Geometry check sheet. Reference: drawing and pictorial views, mm from the part's lowest x, y, z. Round coordinates to 2 decimals unless told otherwise and drop trailing zeros. Order: outer loops, then holes, each group sorted by start corner. A loop starts at its lowest first (then second) coordinate and runs counter-clockwise, first axis right, second up.
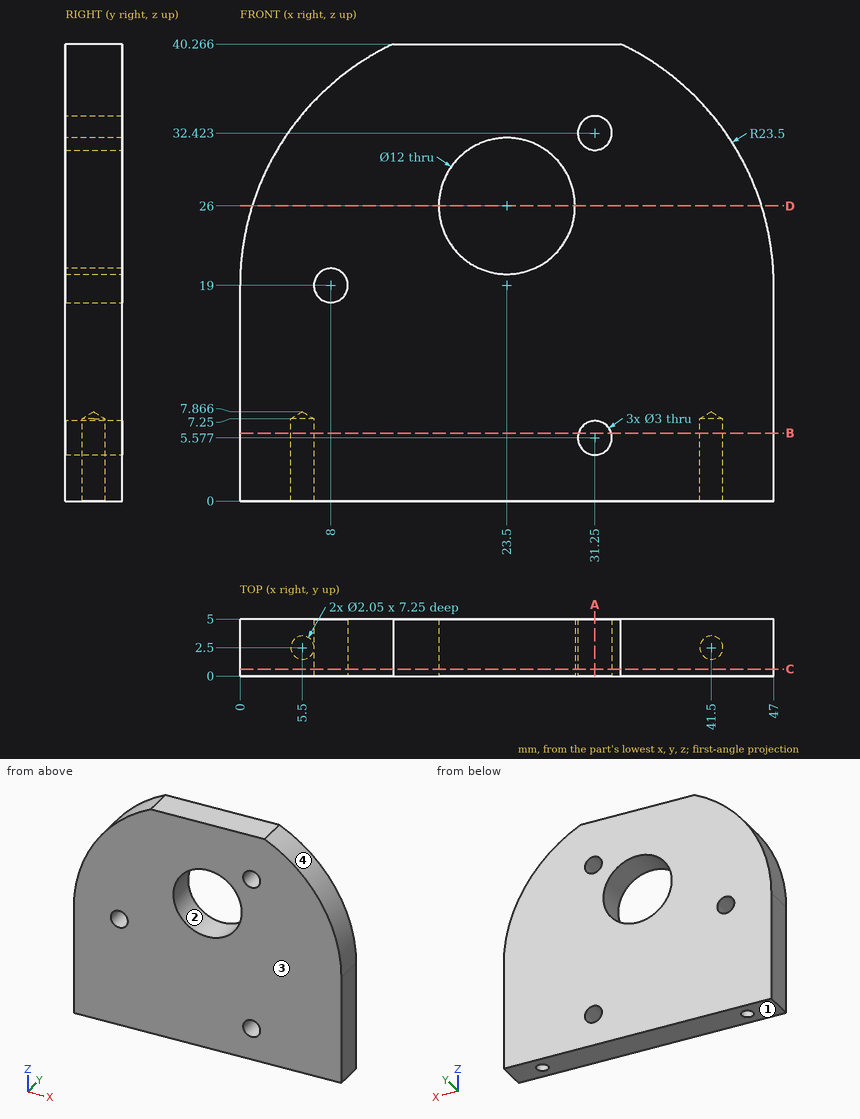
1) Sectioned sample at C-C on y = 0.6. Record the cut outline in (x, z).
2) Sectioned sample at D-D on z = 26. Record the cut outline in (x, y).
3) Sectioned sample at A-A on x = 31.25. Record the cut outline in (y, z).
4) Sectioned sample at B-B on z = 6. Count the separate pieces of the cut face and the enclosed holes in it, then the cut area to 3 significant figures.
5) Scan lines: probe 1 along X at (y, z) = (2.5, 3.5) (1 decimal); probe 2 along X at (y, z) = (3.2, 4); probe 3 along X at (y, z) = (2.5, 5) (1 decimal). Record each from-to range of solid material in increasing order.
6) Draft check along Z on the marked faces 1, 2, 3 and 4. Enter one of: released by +Z, released by -Z, zero draft, split by the parting line, or undercut.
7) Go/stop test with flat-tipped pins: pin 1 Ø3 at (y, z) = (0.5, 13.5) entering from -X; pin 2 Ø1.2 at (x, y) = (41.5, 2.5) entering from -Z (1 decimal); pin 3 Ø1.5 at (y, z) = (3, 21.5) entering from -X (1 decimal). Record where each tip stops, or that it passes through.
Returned:
1. outline: (0, 0) - (47, 0) - (47, 19) arc R23.5 ccw to (33.5, 40.27) - (13.5, 40.27) arc R23.5 ccw to (0, 19) - close; hole circle Ø3 at (8, 19); hole circle Ø12 at (23.5, 26); hole circle Ø3 at (31.25, 5.58); hole circle Ø3 at (31.25, 32.42)
2. outline: (1.07, 0) - (17.5, 0) - (17.5, 5) - (1.07, 5) - close; (29.5, 0) - (45.93, 0) - (45.93, 5) - (29.5, 5) - close
3. outline: (0, 0) - (5, 0) - (5, 4.08) - (0, 4.08) - close; (0, 7.08) - (5, 7.08) - (5, 30.92) - (0, 30.92) - close; (0, 33.92) - (5, 33.92) - (5, 40.27) - (0, 40.27) - close
4. separate pieces: 2
4. enclosed holes: 2
4. area: 214 mm2
5. probe 1: x = 0 to 4.5, 6.5 to 40.5, 42.5 to 47
5. probe 2: x = 0 to 4.75, 6.25 to 40.75, 42.25 to 47
5. probe 3: x = 0 to 4.5, 6.5 to 29.9, 32.6 to 40.5, 42.5 to 47
6. face 1: released by -Z
6. face 2: undercut
6. face 3: zero draft
6. face 4: released by +Z
7. pin 1: stops at x = 0
7. pin 2: stops at z = 7.5
7. pin 3: stops at x = 0.1
